Geometry check sheet. Reference: the model listing, model coordinates, mm. Face numbers are marked on the shaded views. A direction names the side the tool comes from. Round coordinates to 2 decimals unless told otherwise and drop trailing zeros. Loops run counter-clockwise (first coordinate to the right, second up) from the corner with the lowest first, then second, coordinate; pieces in that order, holes last. Notation, with made-up numbers: M 18,44 L 24,44 A14 ccw 24,55 Z; hole C -19.75,-34.75 d3. An arc over 180 degrees is marked long. Use one line per item in the form item = value. Start each with the question number.
1. Cross-section at A-A (y = 56.5). Record the boundary of the cut face in (x, z), then the cut area to 3 significant figures.
2. Material ranges on line 1 (Y direction, x = 30.5, z = 26); line 2 (Y direction, x = 37, z = 42); line 3 (X direction, y = 98, z = -14), recorded low to high.
3. Cross-section at B-B (y = 105). Record the boundary of the cut face in (x, z), then the cut area to 3 significant figures.
4. Draft check along Z on the marked faces 4 and 5. Enter one of: pulls with the +Z half, pulls with the -Z half, needs draft (parallel to the pull), parting line crosses it, or undercut.
5. Go/stop test with flat-tipped pins: pin 1 (1.5 mm diameter, centred on x = -12, z = 8, fed in from +Y); pin 2 (1 mm diameter, centred on x = -5, y = 85, fed in from +Z); pin 3 (8 mm diameter, centred on x = 16.5, z = -33.5, fed in from +Y). Record where each tip stops, or that it passes through.
6. Set-up check for the marked faces 1, 2 and 3: record each of +Z, -Z, +X, -X, +Y, -Y from which the full face is reachable in a straight line by a thin tool's end or side.
Autodesk Fusion 360 part; units mm, degrees
sketch "Esquisse1" plane through (0, 0, 0) normal (0, 0, 1) x (1, 0, 0)
  line L0 (0, 0) -> (-65, 0)
  line L1 (-65, 0) -> (-40, 80)
  line L2 (-40, 80) -> (-79.5161, 101.5285)
  line L3 (-79.5161, 101.5285) -> (-55, 146.5285)
  line L4 (-55, 146.5285) -> (0, 146.8871)
  line L5 (0, 146.8871) -> (0, 0)
  dimension "d1" = 65
  dimension "d2" = 45
  dimension "d3" = 45
  dimension "d4" = 40
  dimension "d5" = 80
  dimension "d6" = 55
revolve "Révolution1" add sketch "Esquisse1" angle 360 about axis through (0, 146.8871, 0) along (0, -1, 0)
shell "Coque1" thickness 2 removed faces 1 at (20.2416, 0, -0.2148)
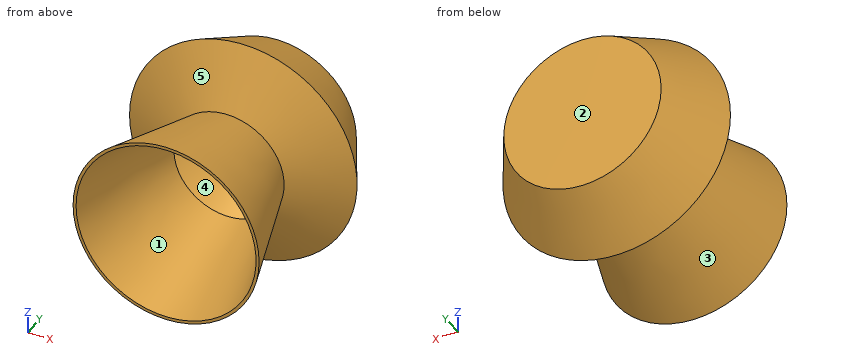
Reported:
q1.outline = C 0,0 d94.69; hole C 0,0 d90.5
q1.area = 610 mm²
q2.line_1 = 73.05 to 79.75, 80.04 to 82.32, 144.63 to 146.63
q2.line_2 = 22.18 to 28.89, 88.7 to 90.98, 140.56 to 144.74
q2.line_3 = -71.69 to -67.42, 67.42 to 71.69
q3.outline = C 0,0 d155.25; hole C 0,0 d150.69
q3.area = 1,090 mm²
q4.face_4 = undercut
q4.face_5 = parting line crosses it
q5.pin_1 = 146.8
q5.pin_2 = 49.85
q5.pin_3 = 146.67
q6.face_1 = -Y
q6.face_2 = +Y
q6.face_3 = none
